Read the model definition and answer for the solid it produces. Units are mm, in the model's axes. Face numbers are marked on the shaded views. Coordinates: 2 decimals unless noted, no trailing zeros. Order: outer loops, then holes, each group sorted by start corner. A loop starts at its lowest first (then second) coordinate and runs counter-clockwise, first axis right, second up.
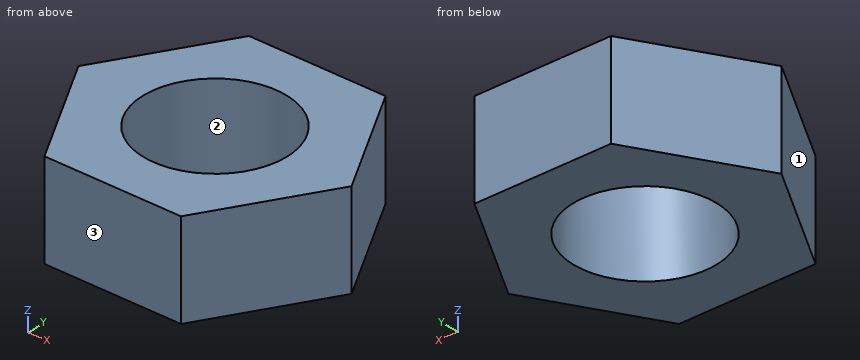
Solid Edge part; units mm, degrees
sketch "Sketch1" plane through (0, 0, 0) normal (0, 0, 1) x (1, 0, 0)
  circle A0 centre (0, 0) radius 6
  line L0 (-5.7741, 10.001) -> (-11.5482, 0)
  line L1 (-11.5482, 0) -> (-5.7741, -10.001)
  line L2 (-5.7741, -10.001) -> (5.7741, -10.001)
  line L3 (5.7741, -10.001) -> (11.5482, 0)
  line L4 (11.5482, 0) -> (5.7741, 10.001)
  line L5 (5.7741, 10.001) -> (-5.7741, 10.001)
extrude "ExtrudedProtrusion_1" add sketch "Sketch1" along normal blind 7 and the other way blind 1
properties material "Steel"
1) Determine the mould class of the marked faces 1, 2 and 3 for opening direction X: pulls with the +X half, pulls with the -X half, needs draft (parallel to the pull), parting line crosses it, or undercut.
A:
face 1: pulls with the -X half
face 2: undercut
face 3: needs draft
2) A cutting plane is placed at B-B, the plane z = 0.75. Determine the outline of the cut face in (x, y).
A:
outline: (-11.55, 0) - (-5.77, -10) - (5.77, -10) - (11.55, 0) - (5.77, 10) - (-5.77, 10) - close; hole circle Ø12 at (0, 0)
3) A cutting plane is placed at A-A, the plane x = 0. Determine the outline of the cut face in (y, z), and give its area (3 significant figures).
A:
outline: (-10, -1) - (-6, -1) - (-6, 7) - (-10, 7) - close; (6, -1) - (10, -1) - (10, 7) - (6, 7) - close
area: 64.0 mm2
4) Flat-ended cylindrical pins translate along their axes: pin 1 Ø1 at (x, z) = (7, 5) entering from +Y; pin 2 Ø4 at (y, z) = (7, 2.5) entering from -X; pin 3 Ø1.5 at (x, z) = (9, 2) entering from -Y. Find the tip coordinate at first contact, or state that the pin passes through.
A:
pin 1: stops at y = 8.74
pin 2: stops at x = -8.66
pin 3: stops at y = -5.71
5) A cutting plane is placed at D-D, the plane x = 7. Determine the outline of the cut face in (y, z), and give its area (3 significant figures).
A:
outline: (-7.88, -1) - (7.88, -1) - (7.88, 7) - (-7.88, 7) - close
area: 126 mm2
6) Straight lines are drawn through the part: line 1 (Y direction, x = 0, z = 2.75); line 2 (Y direction, x = -4.75, z = 0.5); line 3 (X direction, y = -0.5, z = 1). For each, find the intervals that lie inside material, in ascending order.
A:
line 1: y = -10 to -6, 6 to 10
line 2: y = -10 to -3.67, 3.67 to 10
line 3: x = -11.26 to -5.98, 5.98 to 11.26
7) A cutting plane is placed at C-C, the plane y = -2.25. Determine the outline of the cut face in (x, z).
A:
outline: (-10.25, -1) - (-5.56, -1) - (-5.56, 7) - (-10.25, 7) - close; (5.56, -1) - (10.25, -1) - (10.25, 7) - (5.56, 7) - close
